Source: CAD feature listing. Evaluate the final solid. Frame: model axes, mm. Give positions to 0.01 mm unless a question says otherwise; leave off trailing zeros. Order: outer loops, then holes, each group sorted by start corner. A loop starts at its lowest first (then second) coordinate and runs counter-clockwise, first axis right, second up. Notation, with made-up numbers: M -29,67.25 L 8,67.25 A12 ccw 8,75.25 Z; hole C 47,-37.75 d10. An arc over 180 degrees is marked long. Answer as a JSON object with one key per item and string values. Group by question number.
1. Section query B-B (x = -3). Output: boundary loops of the cut face in (y, z), plus the area to 3 significant figures.
2. Pin query (flat end, axial travel): P1, Ø1.2, axis at x = -14, y = 0.5, coming from the +Z side; P2, Ø1, axis at x = -1.5, y = 1, coming from the -Z side. Return the tip coordinate at first contact, or that it passes through.
3. Material intervals for L1, parallel to Z at x = -36.5, y = 1.4; L2, parallel to X at y = 2.7, z = -45.5; L3, parallel to X at y = 2.25, z = -19.5, sorted ascending. Write a range as [from, to].
4. Section query A-A (z = -48.5). Output: boundary loops of the cut face in (x, y), plus the area to 3 significant figures.
5. Section query C-C (y = 0.95). Output: boundary loops of the cut face in (x, z), plus the area to 3 significant figures.
from build123d import *

# Parameters (mm, degrees)
SKETCH_1_W          = 200
SKETCH_1_H          = 115
EXTRUDE_1_DEPTH     = 1.5
SKETCH_2_W          = 203
SKETCH_2_H          = 118
EXTRUDE_2_DEPTH     = 1.5
SKETCH_3_W          = 30
SKETCH_3_H          = 18.47287918
CUT_EXTRUDE_1_DEPTH = 11.5
FILLET_3_R          = 1


with BuildPart() as part:
    # 草图1 → 凸台-拉伸1 (new body)
    with BuildSketch(Plane(origin=(0, 0, 0), x_dir=(1, 0, 0), z_dir=(0, 1, 0))):
        Rectangle(SKETCH_1_W, SKETCH_1_H)
    extrude(amount=EXTRUDE_1_DEPTH)

    # 草图2 → 凸台-拉伸2 (add)
    with BuildSketch(Plane(origin=(0, 1.5, 0), x_dir=(1, 0, 0), z_dir=(0, 1, 0))):
        Rectangle(SKETCH_2_W, SKETCH_2_H)
    extrude(amount=EXTRUDE_2_DEPTH)

    # 草图3 → 切除-拉伸1 (cut)
    with BuildSketch(Plane.XZ):
        with Locations((0, -51.38442851)):
            Rectangle(SKETCH_3_W, SKETCH_3_H)
    extrude(amount=-CUT_EXTRUDE_1_DEPTH, mode=Mode.SUBTRACT)

    # 圆角3
    fillet_3_edges = [part.edges().sort_by_distance(p)[0] for p in [
        (101.5, 3, 0),
        (58.25, 3, -59),
        (-101.5, 3, 0),
        (0, 3, 59),
        (-58.25, 3, -59),
        (0, 3, -42.14798892),
        (15, 3, -50.57399446),
        (-15, 3, -50.57399446),
    ]]
    fillet(fillet_3_edges, radius=FILLET_3_R)


solid = part.part
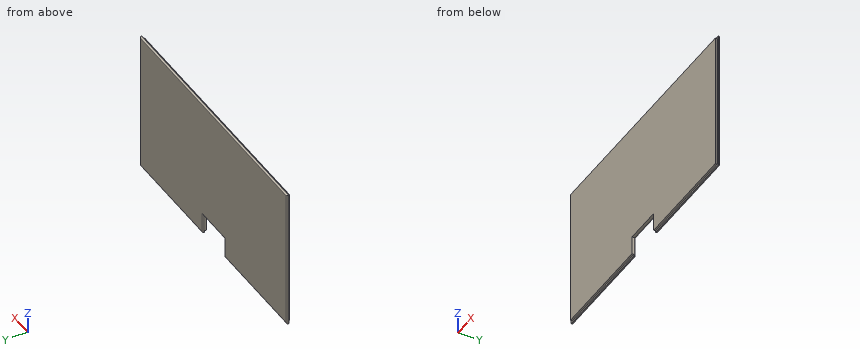
Answer sheet:
{
 "1": {"outline": "M 0,-42.15 L 2,-42.15 A1 ccw 3,-41.15 L 3,58 A1 ccw 2,59 L 1.5,59 L 1.5,57.5 L 0,57.5 Z", "area": "301 mm^2"},
 "2": {"P1": "z = 57.5", "P2": "z = -42.15"},
 "3": {"L1": "[-57.5, 57.5]", "L2": "[-101.21, -15.29], [15.29, 101.21]", "L3": "[-101.47, 101.47]"},
 "4": {"outline": "M -101.5,1.5 L -100,1.5 L -100,0 L -15,0 L -15,2 A1 ccw -16,3 L -100.5,3 A1 ccw -101.5,2 Z; M 15,0 L 100,0 L 100,1.5 L 101.5,1.5 L 101.5,2 A1 ccw 100.5,3 L 16,3 A1 ccw 15,2 Z", "area": "514 mm^2"},
 "5": {"outline": "M -100,-57.5 L -15,-57.5 L -15,-42.15 L 15,-42.15 L 15,-57.5 L 100,-57.5 L 100,57.5 L -100,57.5 Z", "area": "22,500 mm^2"}
}
